Could you check a few things on this model? Use its own coordinates, in mm. Coordinates: 2 decimals unless noted, no trailing zeros. Loops run counter-clockwise (first coordinate to the right, second up) from the corner with the lowest first, then second, coordinate; pieces in that order, holes last.
1) Imagine slicing it at A-A on y = 4. Please give me the cut outline in (x, z).
2) Imagine slicing it at C-C on x = 5. Please give me the cut outline in (y, z), plus the area to 3 significant figures.
3) Imagine slicing it at B-B on z = -2.1. Please give me the cut outline in (x, y), plus the area to 3 significant figures.
4) Will these pins go through, and if not, where does the flat tip stop? P1, Ø1.5, axis at x = 5, z = -0.5, coming from the +Y side; P2, Ø2, axis at x = 6.5, z = -2.5, coming from the +Y side.
5) Imagine slicing it at D-D on y = 6.25. Please give me the cut outline in (x, z).
6) Thinking about a two-plate mould opening in X: for faces 1 (the face through (4, 2, -4)), 2 (the face through (1.918, 8.188, -1.972)), 3 (the face through (6.1, 8.19, -1.97)), 4 (the face through (7.966, 5.519, -1.972)), which applies, released by +X, released by -X, zero draft, split by the parting line, or undercut?
7) If I drill on line 1 along Y through (x, z) = (4.75, -1.5); line 2 along X through (y, z) = (5.5, -0.5); line 3 along X through (y, z) = (7.5, -3), over which ranges is the centre line in solid material (lowest first)?
```python
from build123d import *

# Parameters (mm, degrees)
SKETCH_1_W      = 8
SKETCH_1_H      = 4
EXTRUDE_1_DEPTH = 1
EXTRUDE_2_DEPTH = 4
SKETCH_1_2_W    = 8
SKETCH_1_2_H    = 4
EXTRUDE_3_DEPTH = 2
FILLET_1_R      = 0.5


with BuildPart() as part:
    # Sketch 1 → Extrude 1 (new body)
    with BuildSketch(Plane(origin=(0, 0, 0), x_dir=(1, 0, 0), z_dir=(0, 1, 0))):
        with Locations((4, 2)):
            Rectangle(SKETCH_1_W, SKETCH_1_H)
    extrude(amount=EXTRUDE_1_DEPTH)



with BuildPart() as body_2:
    # Sketch 2 → Extrude 2 (new body)
    with BuildSketch(Plane.XY):
        with BuildLine():
            ThreePointArc((5.779316158, 7.096791361), (6.581537937, 4.052285972), (4, 2.25))
            Line((4, 2.25), (4, 1))
            ThreePointArc((4, 1), (7.756805699, 3.626533239), (6.579923877, 8.056794529))
            ThreePointArc((6.579923877, 8.056794529), (6.089593434, 8.189308732), (5.673320053, 7.898275349))
            Line((5.673320053, 7.898275349), (5.64791535, 7.854273112))
            ThreePointArc((5.64791535, 7.854273112), (5.57635944, 7.451722303), (5.779316158, 7.096791361))
        make_face()
        with BuildLine():
            ThreePointArc((2.220683842, 7.096791361), (2.42364056, 7.451722303), (2.35208465, 7.854273112))
            Line((2.35208465, 7.854273112), (2.326679947, 7.898275349))
            ThreePointArc((2.326679947, 7.898275349), (1.910406566, 8.189308732), (1.420076123, 8.056794529))
            ThreePointArc((1.420076123, 8.056794529), (0.243194301, 3.626533239), (4, 1))
            Line((4, 1), (4, 2.25))
            ThreePointArc((4, 2.25), (1.418462063, 4.052285972), (2.220683842, 7.096791361))
        make_face()
    extrude(amount=-EXTRUDE_2_DEPTH)


with BuildPart() as part_1:
    add(part.part)

    add(body_2.part)  # Extrude 3 merges body 2
    # Sketch 1_2 → Extrude 3 (add)
    with BuildSketch(Plane(origin=(0, 0, 0), x_dir=(1, 0, 0), z_dir=(0, 1, 0))):
        with Locations((4, 2)):
            Rectangle(SKETCH_1_2_W, SKETCH_1_2_H)
    extrude(amount=EXTRUDE_3_DEPTH)

    # Fillet 1
    fillet_1_edges = [part_1.edges().sort_by_distance(p)[0] for p in [
        (1.354248689, 2, -2),
        (6.645751311, 2, -2),
    ]]
    fillet(fillet_1_edges, radius=FILLET_1_R)


solid = part_1.part
```
Filled in:
1. outline: (0.13, -4) - (1.44, -4) - (1.44, 0) - (0.13, 0) - close; (6.56, -4) - (7.87, -4) - (7.87, 0) - (6.56, 0) - close
2. outline: (0, -4) - (2.44, -4) - (2.44, 0) - (0, 0) - close
2. area: 9.75 mm2
3. outline: (0, 0) - (8, 0) - (8, 2) - (7.74, 2) arc R0.5 cw to (7.33, 2.78) arc R4 ccw to (6.58, 8.06) arc R0.6 ccw to (5.67, 7.9) - (5.65, 7.85) arc R0.6 ccw to (5.78, 7.1) arc R2.75 cw (long way) to (2.22, 7.1) arc R0.6 ccw to (2.35, 7.85) - (2.33, 7.9) arc R0.6 ccw to (1.42, 8.06) arc R4 ccw to (0.67, 2.78) arc R0.5 cw to (0.26, 2) - (0, 2) - close
3. area: 34.6 mm2
4. P1: stops at y = 8
4. P2: stops at y = 8.2
5. outline: (0.2, -4) - (1.55, -4) - (1.55, 0) - (0.2, 0) - close; (6.45, -4) - (7.8, -4) - (7.8, 0) - (6.45, 0) - close
6. face 1: zero draft
6. face 2: undercut
6. face 3: undercut
6. face 4: released by +X
7. line 1: y = 0 to 2.35
7. line 2: x = 0.03 to 1.3, 6.7 to 7.97
7. line 3: x = 0.88 to 2.43, 5.57 to 7.12
